Here's how the part is built. I have some questions about the finished solid (model axes, mm). A direction names the side the tool comes from. Coordinates: 2 decimals unless noted, no trailing zeros. Loops run counter-clockwise (first coordinate to the right, second up) from the corner with the lowest first, then second, coordinate; pieces in that order, holes last. Notation, with made-up numbers: (38.5, -26.75) - (92.5, -26.75) arc R10 ccw to (92.5, -17.75) - close; hole circle Ø3 at (60, 31). An arc over 180 degrees is marked (long way). Use a Markdown table: item, result.
```python
from build123d import *

# Parameters (mm, degrees)
SKETCH1_R                      = 8.89
BOSS_EXTRUDE1_DEPTH            = 6.35
SKETCH2_R                      = 9.525
CUT_EXTRUDE1_DEPTH             = 4.7625
SKETCH3_R                      = 9.525
SKETCH3_R_2                    = 8.255
BOSS_EXTRUDE2_DEPTH            = 4.75996
CHAMFER1_SIZE                  = 0.254
SKETCH4_R                      = 6.985
SKETCH4_R_2                    = 6.35
BOSS_EXTRUDE3_DEPTH            = 4.75996
CHAMFER2_SIZE                  = 0.254
SKETCH5_R                      = 8.255
SKETCH5_R_2                    = 6.985
BOSS_EXTRUDE4_DEPTH            = 4.2545
F_6_32_TAPPED_HOLE1_AT_2_COUNT = 2
F_6_32_TAPPED_HOLE1_AT_2_PITCH = 26.940768363


with BuildPart() as part:
    # Sketch1 → Boss-Extrude1 (new body)
    with BuildSketch(Plane(origin=(0, 0, 0), x_dir=(1, 0, 0), z_dir=(0, 1, 0))):
        with BuildLine():
            Line((-16.764, -16.51), (-7.62, -16.51))
            Line((-7.62, -16.51), (-7.62, -14.9479))
            ThreePointArc((-7.62, -14.9479), (-7.155032015, -13.825367985), (-6.0325, -13.3604))
            Line((-6.0325, -13.3604), (6.0325, -13.3604))
            ThreePointArc((6.0325, -13.3604), (7.155032015, -13.825367985), (7.62, -14.9479))
            Line((7.62, -14.9479), (7.62, -16.51))
            Line((7.62, -16.51), (16.764, -16.51))
            Line((16.764, -16.51), (16.764, -10.4267))
            Line((16.764, -10.4267), (15.1765, -10.4267))
            ThreePointArc((15.1765, -10.4267), (14.053967985, -9.961732015), (13.589, -8.8392))
            Line((13.589, -8.8392), (13.589, 8.8392))
            ThreePointArc((13.589, 8.8392), (14.053967985, 9.961732015), (15.1765, 10.4267))
            Line((15.1765, 10.4267), (16.764, 10.4267))
            Line((16.764, 10.4267), (16.764, 16.51))
            Line((16.764, 16.51), (7.62, 16.51))
            Line((7.62, 16.51), (7.62, 14.9479))
            ThreePointArc((7.62, 14.9479), (7.155032015, 13.825367985), (6.0325, 13.3604))
            Line((6.0325, 13.3604), (-6.0325, 13.3604))
            ThreePointArc((-6.0325, 13.3604), (-7.155032015, 13.825367985), (-7.62, 14.9479))
            Line((-7.62, 14.9479), (-7.62, 16.51))
            Line((-7.62, 16.51), (-16.764, 16.51))
            Line((-16.764, 16.51), (-16.764, 10.4267))
            Line((-16.764, 10.4267), (-15.1765, 10.4267))
            ThreePointArc((-15.1765, 10.4267), (-14.053967985, 9.961732015), (-13.589, 8.8392))
            Line((-13.589, 8.8392), (-13.589, -8.8392))
            ThreePointArc((-13.589, -8.8392), (-14.053967985, -9.961732015), (-15.1765, -10.4267))
            Line((-15.1765, -10.4267), (-16.764, -10.4267))
            Line((-16.764, -10.4267), (-16.764, -16.51))
        make_face()
        Circle(SKETCH1_R, mode=Mode.SUBTRACT)
    extrude(amount=BOSS_EXTRUDE1_DEPTH)

    # Sketch2 → Cut-Extrude1 (cut)
    with BuildSketch(Plane(origin=(0, 6.35, 0), x_dir=(1, 0, 0), z_dir=(0, 1, 0))):
        Circle(SKETCH2_R)
    extrude(amount=-CUT_EXTRUDE1_DEPTH, mode=Mode.SUBTRACT)

    # Sketch3 → Boss-Extrude2 (add)
    with BuildSketch(Plane(origin=(0, 1.5875, 0), x_dir=(-1, 0, 0), z_dir=(0, 1, 0))):
        Circle(SKETCH3_R)
        Circle(SKETCH3_R_2, mode=Mode.SUBTRACT)
    extrude(amount=BOSS_EXTRUDE2_DEPTH)

    # Chamfer1
    chamfer1_edges = [part.edges().sort_by_distance(p)[0] for p in [
        (8.255, 1.5875, 0),
        (8.255, 6.34746, 0),
    ]]
    chamfer(chamfer1_edges, length=CHAMFER1_SIZE)



with BuildPart() as body_2:
    # Sketch4 → Boss-Extrude3 (new body)
    with BuildSketch(Plane(origin=(0, 1.5875, 0), x_dir=(-1, 0, 0), z_dir=(0, 1, 0))):
        Circle(SKETCH4_R)
        Circle(SKETCH4_R_2, mode=Mode.SUBTRACT)
    extrude(amount=BOSS_EXTRUDE3_DEPTH)

    # Chamfer2
    chamfer2_edges = [body_2.edges().sort_by_distance(p)[0] for p in [
        (6.985, 1.5875, 0),
        (6.985, 6.34746, 0),
    ]]
    chamfer(chamfer2_edges, length=CHAMFER2_SIZE)


with BuildPart() as part_1:
    add(part.part)

    add(body_2.part)  # Boss-Extrude4 merges body 2
    # Sketch5 → Boss-Extrude4 (add)
    with BuildSketch(Plane(origin=(0, 6.09346, 0), x_dir=(-1, 0, 0), z_dir=(0, 1, 0))):
        Circle(SKETCH5_R)
        Circle(SKETCH5_R_2, mode=Mode.SUBTRACT)
    extrude(amount=-BOSS_EXTRUDE4_DEPTH)

    # Sketch8 → #6-32 Tapped Hole1 (revolve, cut)
    with BuildSketch(Plane(origin=(-16.764, 3.175, -13.470384182), x_dir=(0, 0, 1), z_dir=(0, 1, 0))):
        Polygon((0, 0), (0, 8.76289403), (1.35255, 7.9502), (1.35255, 7.0104), (1.7526, 7.0104), (1.7526, 0), align=None)
    f_6_32_tapped_hole1 = revolve(axis=Axis((-23.114, 3.175, -13.470384182), (1, 0, 0)), mode=Mode.SUBTRACT)

    # #6-32 Tapped Hole1 at 2: #6-32 Tapped Hole1 ×2
    with Locations(*[(0, 0, i * F_6_32_TAPPED_HOLE1_AT_2_PITCH) for i in range(1, F_6_32_TAPPED_HOLE1_AT_2_COUNT)]):
        add(f_6_32_tapped_hole1, mode=Mode.SUBTRACT)

    # Mirror1: #6-32 Tapped Hole1 across plane
    add(f_6_32_tapped_hole1.mirror(Plane(origin=(0, 0, 0), x_dir=(0, 0, 1), z_dir=(1, 0, 0))), mode=Mode.SUBTRACT)

    # Mirror1 copy 1 sketch → Mirror1 copy 1 (revolve, cut)
    with BuildSketch(Plane(origin=(16.764, 3.175, 13.470384182), x_dir=(0, 0, 1), z_dir=(0, 1, 0))):
        Polygon((0, 0), (0, -8.76289403), (1.35255, -7.9502), (1.35255, -7.0104), (1.7526, -7.0104), (1.7526, 0), align=None)
    revolve(axis=Axis((23.114, 3.175, 13.470384182), (1, 0, 0)), mode=Mode.SUBTRACT)


solid = part_1.part
```
Q1. If we mould it in two halves opening along Z, with no side actions, what happens to faces 6 (the face through (-12, 3, 16.51)), 7 (the face through (7.62, 3, -16)), 8 (the face through (-2.5, 1.588, -6))? For each: pulls with the +Z half, pulls with the -Z half, needs draft (parallel to the pull), parting line crosses it, or undercut.
Check values:
| item | result |
|---|---|
| face 6 | pulls with the +Z half |
| face 7 | needs draft |
| face 8 | undercut |
Q2. Please list where these lines run through material, in increasing order: L1, parallel to Z at x = 2, y = 3.25; L2, parallel to X at y = 4.25, z = 15.5; L3, parallel to Z at x = 0, y = 1.8. Write a range as from..to.
Check values:
| item | result |
|---|---|
| L1 | -13.36..-6.03, 6.03..13.36 |
| L2 | -16.76..-7.62, 7.62..16.76 |
| L3 | -13.36..-8.3, -6.94..-6.35, 6.35..6.94, 8.3..13.36 |
Q3. I want a section at B-B, the plane x = 10.5. Write out the boundary of the cut face in (y, z) (3 decimals).
Check values:
| item | result |
|---|---|
| outline | (0, -16.51) - (6.35, -16.51) - (6.35, 16.51) - (0, 16.51) - close; hole circle Ø3.505 at (3.175, -13.47); hole circle Ø3.505 at (3.175, 13.47) |
Q4. Will these pins go through, and if not, where does the flat tip stop? P1, Ø3, axis at y = 5.5, z = -1, coming from the +X side; P2, Ø6.5, axis at x = 0.5, z = 1, coming from the -Y side; P3, Ø1, axis at x = -1.5, y = 5.5, coming from the +Z side; P4, Ø1.5, axis at x = -6.5, y = 2, coming from the +Z side.
Check values:
| item | result |
|---|---|
| P1 | x = 13.59 |
| P2 | through |
| P3 | z = 13.36 |
| P4 | z = 13.93 |
Q5. Which directions (+Z, -Z, +X, -X, +Y, -Y) give clear straight access to the entire face, cutting with the end or side of a thin tool? Please do faces 1 (the face through (9.29, 3.12, 12.12)), 2 (the face through (-7.14, 3.13, -13.81)), 3 (the face through (-13.589, 3, 0)), 4 (the face through (-7.17, 3.13, 13.84)), 5 (the face through (-13.31, 3.1, 11.72)).
Check values:
| item | result |
|---|---|
| face 1 | +X |
| face 2 | -Z, +Y, -Y |
| face 3 | -X, +Y, -Y |
| face 4 | +Z, +Y, -Y |
| face 5 | -X |
